Could you check a few things on this model? Use its own coordinates, in mm. Round coordinates to 2 decimals unless told otherwise and drop trailing zeros. Loops run counter-clockwise (first coordinate to the right, second up) from the corner with the lowest first, then second, coordinate; pieces in that order, holes last.
from build123d import *

# Parameters (mm, degrees)
SKETCH1_W           = 355.6
SKETCH1_H           = 114.3
BOSS_EXTRUDE1_DEPTH = 6.35
SKETCH3_R           = 3.175
CUT_EXTRUDE1_DEPTH  = 6.35


with BuildPart() as part:
    # Sketch1 → Boss-Extrude1 (new body)
    with BuildSketch(Plane.XY):
        Rectangle(SKETCH1_W, SKETCH1_H)
    extrude(amount=BOSS_EXTRUDE1_DEPTH)

    # Sketch3 → Cut-Extrude1 (cut)
    with BuildSketch(Plane.XY.offset(6.35)):
        with Locations((-60.325, 0)):
            Circle(SKETCH3_R)
        Circle(SKETCH3_R)
        with Locations((-150.749, 20)):
            Circle(SKETCH3_R)
    cut_extrude1 = extrude(amount=-CUT_EXTRUDE1_DEPTH, mode=Mode.SUBTRACT)

    # Mirror3: Cut-Extrude1 across plane
    add(cut_extrude1.mirror(Plane(origin=(0, 0, 0), x_dir=(0, 0, 1), z_dir=(1, 0, 0))), mode=Mode.SUBTRACT)


solid = part.part
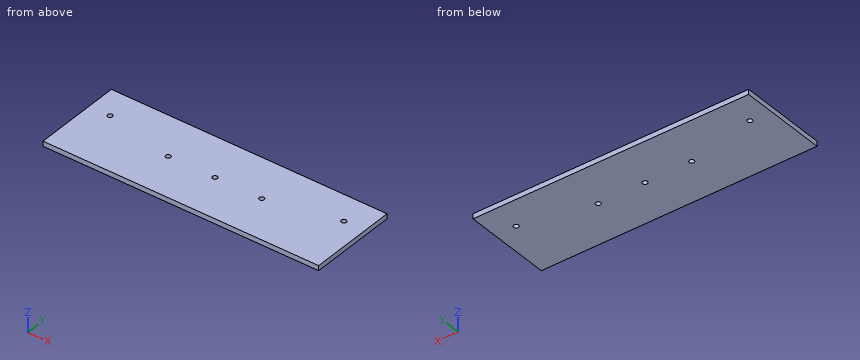
Item 1: If we section it at B-B, the plane x = 0: Please give me the cut outline in (y, z) (3 decimals), then the cut area to 3 significant figures.
Results list:
outline: (-57.15, 0) - (-3.175, 0) - (-3.175, 6.35) - (-57.15, 6.35) - close; (3.175, 0) - (57.15, 0) - (57.15, 6.35) - (3.175, 6.35) - close
area: 685 mm2
Item 2: If I drill on line 1 along Y through (x, z) = (0, 2.5) (3 decimals); line 2 along Y through (x, z) = (-153, 3), over which ranges is the centre line in solid material (lowest first)?
Results list:
line 1: y = -57.15 to -3.175, 3.175 to 57.15
line 2: y = -57.15 to 17.76, 22.24 to 57.15
Item 3: If we section it at A-A, the plane y = 20: Please give me the cut outline in (x, z).
Results list:
outline: (-177.8, 0) - (-153.92, 0) - (-153.92, 6.35) - (-177.8, 6.35) - close; (-147.57, 0) - (147.57, 0) - (147.57, 6.35) - (-147.57, 6.35) - close; (153.92, 0) - (177.8, 0) - (177.8, 6.35) - (153.92, 6.35) - close
